Part model, mm, in its own coordinate system. A direction names the side the tool comes from. Give positions to 0.01 mm unless a question says otherwise; leave off trailing zeros. Order: outer loops, then holes, each group sorted by start corner. A loop starts at its lowest first (then second) coordinate and runs counter-clockwise, first axis right, second up. Notation, with made-up numbers: (22, 2) - (48, 2) arc R24 ccw to (48, 27) - close; hole circle Ø11 at (17, 7). An arc over 180 degrees is marked (long way). One line per item, written item: value.
Autodesk Inventor part; units mm, degrees
ref_plane "YZ Plane" through (0, 0, 0) normal (1, 0, 0) x (0, 1, 0)
ref_plane "XZ Plane" through (0, 0, 0) normal (0, 1, 0) x (-1, 0, 0)
ref_plane "XY Plane" through (0, 0, 0) normal (0, 0, 1) x (1, 0, 0)
sketch "Sketch5" plane through (0, 0, 0) normal (1, 0, 0) x (0, 1, 0)
  line L0 (-38.1, 50.8) -> (38.1, 50.8)
  line L1 (50.8, 38.1) -> (50.8, -38.1)
  line L2 (38.1, -50.8) -> (-38.1, -50.8)
  line L3 (-50.8, -38.1) -> (-50.8, 38.1)
  line L4 (-50.8, 50.8) -> (50.8, -50.8) construction
  line L5 (50.8, 50.8) -> (-50.8, -50.8) construction
  arc A0 (50.8, 38.1) -> (38.1, 50.8) centre (38.1, 38.1) ccw
  arc A1 (38.1, -50.8) -> (50.8, -38.1) centre (38.1, -38.1) ccw
  arc A2 (-50.8, -38.1) -> (-38.1, -50.8) centre (-38.1, -38.1) ccw
  arc A3 (-38.1, 50.8) -> (-50.8, 38.1) centre (-38.1, 38.1) ccw
  line L6 (44.45, -38.1) -> (44.45, 38.1)
  arc A4 (44.45, 38.1) -> (38.1, 44.45) centre (38.1, 38.1) ccw
  line L7 (38.1, 44.45) -> (-38.1, 44.45)
  arc A5 (-38.1, 44.45) -> (-44.45, 38.1) centre (-38.1, 38.1) ccw
  line L8 (-44.45, 38.1) -> (-44.45, -38.1)
  arc A6 (-44.45, -38.1) -> (-38.1, -44.45) centre (-38.1, -38.1) ccw
  line L9 (-38.1, -44.45) -> (38.1, -44.45)
  arc A7 (38.1, -44.45) -> (44.45, -38.1) centre (38.1, -38.1) ccw
  point P0 (0, 0)
  dimension "d6" = 101.6
  dimension "d7" = 101.6
  dimension "d8" = 12.7
  dimension "d9" = 6.35
extrude "Extrusion4" add sketch "Sketch5" along normal mid plane 1111.25
sketch "Sketch9" plane through (-555.625, 50.8, 38.1) normal (0, 1, 0) x (1, 0, 0)
  line L0 (0, 38.1) -> (1111.25, 38.1) construction
  line L1 (1111.25, 0) -> (1111.25, 76.2)
  circle A0 centre (76.2, 38.1) radius 14.2875
  line L2 (0, 0) -> (0, 76.2)
  circle A1 centre (1035.05, 38.1) radius 14.2875
  point P0 (555.625, 38.1)
  dimension "d30" = 28.575
  dimension "d31" = 76.2
  dimension "d32" = 76.2
extrude "Extrusion8" cut sketch "Sketch9" against normal blind 382.5875
properties part number "Model-4_Base Tube-1" material "SS304"
1) Slice it at C-C on z = 0. Count the separate pieces of the cut face and the enclosed holes in it, then the cut area to 3 significant figures.
Answer:
separate pieces: 6
enclosed holes: 0
area: 13,400 mm2
2) Drop a flat-ended pin along its axis: P1, Ø17, axis at x = -479.425, z = 0, coming from the +Y side. Give the stop position or say it passes through.
Answer:
P1: passes through
3) Wall check: line 1 along X through (y, z) = (46, 0) (1 decimal); line 2 along Y through (x, z) = (-452.5, 22.5). Give the ranges that are in metal, low to high. Write a range as [from, to].
Answer:
line 1: x = [-555.6, -493.7], [-465.1, 465.1], [493.7, 555.6]
line 2: y = [-50.8, -44.45], [44.45, 50.8]
4) Slice it at A-A on x = -305. Write the cut outline in (y, z), then the cut area to 3 significant figures.
Answer:
outline: (-50.8, -38.1) arc R12.7 ccw to (-38.1, -50.8) - (38.1, -50.8) arc R12.7 ccw to (50.8, -38.1) - (50.8, 38.1) arc R12.7 ccw to (38.1, 50.8) - (-38.1, 50.8) arc R12.7 ccw to (-50.8, 38.1) - close; hole (-44.45, -38.1) arc R6.35 ccw to (-38.1, -44.45) - (38.1, -44.45) arc R6.35 ccw to (44.45, -38.1) - (44.45, 38.1) arc R6.35 ccw to (38.1, 44.45) - (-38.1, 44.45) arc R6.35 ccw to (-44.45, 38.1) - close
area: 2,320 mm2
5) Two-plate mould, pull along X, no slides. Class faces 3 (the face through (-493.7, 47.7, -0.6)), 4 (the face through (-555.625, 0, -45)), 5 (the face through (465.15, 47.67, -0.63)), 6 (the face through (-8, 1, 44.45)): pulls with the +X half, pulls with the -X half, needs draft (parallel to the pull), parting line crosses it, or undercut.
Answer:
face 3: undercut
face 4: pulls with the -X half
face 5: undercut
face 6: needs draft
6) Slice it at B-B on y = -23. Write the cut outline in (x, z) (3 decimals), then the cut area to 3 significant figures.
Answer:
outline: (-555.625, -50.8) - (555.625, -50.8) - (555.625, -44.45) - (-555.625, -44.45) - close; (-555.625, 44.45) - (555.625, 44.45) - (555.625, 50.8) - (-555.625, 50.8) - close
area: 14,100 mm2
7) Which spindle directions (+Z, -Z, +X, -X, +Y, -Y) get a long thin tool onto all of the face, cutting with end or side? Do faces 1 (the face through (-8, 44.45, -1)), 2 (the face through (-493.7, -47.6, -0.6)). Say none if no direction does.
Answer:
face 1: +X, -X
face 2: +Y, -Y
